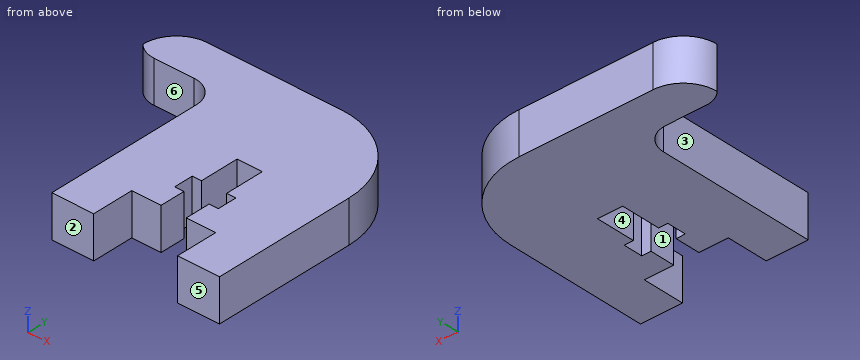
from build123d import *

# Parameters (mm, degrees)
BOSS_EXTRUDE1_DEPTH = 5
FILLET1_R           = 10
FILLET2_R           = 4
FILLET3_R           = 3


with BuildPart() as part:
    # Sketch1 → Boss-Extrude1 (new body)
    with BuildSketch(Plane.XY):
        Polygon((-24.942517195, 5), (-28.442517195, 5), (-28.442517195, 0), (-33.442517195, 0), (-33.442517195, 5), (-33.442517195, 22), (-43.442517195, 22), (-43.442517195, 27), (-13.442517195, 27), (-13.442517195, 5), (-13.442517195, 0), (-18.442517195, 0), (-18.442517195, 5), (-21.942517195, 5), (-21.942517195, 8), (-20.842517195, 8), (-20.842517195, 10.3), (-21.942517195, 10.3), (-21.942517195, 15), (-24.942517195, 15), (-24.942517195, 10.3), (-26.042517195, 10.3), (-26.042517195, 8), (-24.942517195, 8), align=None)
    extrude(amount=BOSS_EXTRUDE1_DEPTH)

    # Fillet1
    fillet1_edges = [part.edges().sort_by_distance(p)[0] for p in [
        (-13.442517195, 27, 2.5),
    ]]
    fillet(fillet1_edges, radius=FILLET1_R)

    # Fillet2
    fillet2_edges = [part.edges().sort_by_distance(p)[0] for p in [
        (-43.442517195, 27, 2.5),
    ]]
    fillet(fillet2_edges, radius=FILLET2_R)

    # Fillet3
    # the kernel refuses this fillet: 3 mm, written as the material it adds along each edge
    with BuildSketch(Plane(origin=(-33.442517195, 22, 0), x_dir=(-1, 0, 0), z_dir=(0, 0, 1))) as fillet3_piece_1:
        with BuildLine():
            CenterArc((FILLET3_R, FILLET3_R), FILLET3_R, 180, 90)
            Line((0, FILLET3_R), (0, 0))
            Line((0, 0), (FILLET3_R, 0))
        make_face()
    extrude(amount=5)
    # the kernel refuses this fillet: 3 mm, written as the material it takes off along each edge
    with BuildSketch(Plane(origin=(-43.442517195, 22, -5.590169944), x_dir=(0, 1, 0), z_dir=(0, 0, 1))) as fillet3_2_piece_1:
        with BuildLine():
            CenterArc((3, -2.236067977), FILLET3_R, 131.810314896, 48.189685104)
            Line((0, -2.236067977), (0, 0))
            Line((0, 0), (1, 0))
        make_face()
    extrude(amount=16.180339887, mode=Mode.SUBTRACT)


solid = part.part
Could you check a few things on this model? Use its own coordinates, in mm. Face numbers are marked on the shaded views. A direction names the side the tool comes from. Round coordinates to 2 decimals unless told otherwise and drop trailing zeros. Order: outer loops, then holes, each group sorted by start corner. A loop starts at its lowest first (then second) coordinate and runs counter-clockwise, first axis right, second up. Notation, with made-up numbers: M -22.75,-3.5 L 34.25,-3.5 A31 cw 34.25,29.5 Z; hole C 42,-6.75 d2. An arc over 180 degrees is marked long. One line per item, written item: value.
(1) Imagine slicing it at D-D (x = -28). Write out the boundary of the cut face in (y, z), and give its area (3 significant figures).
Ans:
outline: M 5,0 L 27,0 L 27,5 L 5,5 Z
area: 110 mm^2
(2) I'm going to push flat-ended pins straight in: P1, Ø3, axis at x = -29.5, y = 2.5, coming from the -Z side; P2, Ø1, axis at x = -19.5, z = 2.5, coming from the -Y side; P3, Ø0.6, axis at x = -21, z = 1.5, coming from the +Y side; P4, Ø0.9, axis at x = -23.5, z = 1.5, coming from the -Y side. Where does each tip first touch, or does it pass through?
Ans:
P1: stops at z = 0
P2: stops at y = 5
P3: stops at y = 26.77
P4: stops at y = 15
(3) If we mould it in two halves opening along X, with no side actions, what happens to the marked faces 1, 2 and 3? For each: released by +X, released by -X, zero draft, split by the parting line, or undercut.
Ans:
face 1: undercut
face 2: zero draft
face 3: released by -X
(4) Imagine slicing it at A-A (y = 7). Write out the boundary of the cut face in (x, z).
Ans:
outline: M -33.44,0 L -24.94,0 L -24.94,5 L -33.44,5 Z; M -21.94,0 L -13.44,0 L -13.44,5 L -21.94,5 Z
(5) Imagine slicing it at C-C (z = 4.35). Write out the boundary of the cut face in (x, y).
Ans:
outline: M -43.44,23 A3 ccw -41.21,22 L -36.44,22 A3 cw -33.44,19 L -33.44,0 L -28.44,0 L -28.44,5 L -24.94,5 L -24.94,8 L -26.04,8 L -26.04,10.3 L -24.94,10.3 L -24.94,15 L -21.94,15 L -21.94,10.3 L -20.84,10.3 L -20.84,8 L -21.94,8 L -21.94,5 L -18.44,5 L -18.44,0 L -13.44,0 L -13.44,17 A10 ccw -23.44,27 L -39.44,27 A4 ccw Z
(6) Which directions (+Z, -Z, +X, -X, +Y, -Y) give clear straight access to the entire face, cutting with the end or side of a thin tool? Please do the marked faces 4, 5 and 6.
Ans:
face 4: +Z, -Z, -Y
face 5: +Z, -Z, +X, -X, -Y
face 6: +Z, -Z, -X, -Y
(7) Imagine slicing it at B-B (x = -21.5). Write out the boundary of the cut face in (y, z), and give its area (3 significant figures).
Ans:
outline: M 5,0 L 8,0 L 8,5 L 5,5 Z; M 10.3,0 L 26.81,0 L 26.81,5 L 10.3,5 Z
area: 97.5 mm^2
(8) I need wall thicknesses on line 1 along X through (y, z) = (11.5, 2); line 2 along X through (y, z) = (3.75, 3.35); line 3 along Y through (x, z) = (-21.5, 2.5). Which ranges of each line are inside material? Lowest first, please. Write a range as from..to.
Ans:
line 1: x = -33.44..-24.94, -21.94..-13.44
line 2: x = -33.44..-28.44, -18.44..-13.44
line 3: y = 5..8, 10.3..26.81
